Autodesk Inventor part; units mm, degrees
ref_plane "YZ Plane" through (0, 0, 0) normal (1, 0, 0) x (0, 1, 0)
ref_plane "XZ Plane" through (0, 0, 0) normal (0, 1, 0) x (-1, 0, 0)
ref_plane "XY Plane" through (0, 0, 0) normal (0, 0, 1) x (1, 0, 0)
sketch "Sketch1" plane through (0, 0, 0) normal (0, 1, 0) x (-1, 0, 0)
  point P0 (0, 0)
sketch "Sketch2" plane through (0, 0, 0) normal (0, 1, 0) x (-1, 0, 0)
  line L0 (70, -12) -> (70, -66)
  line L1 (70, -66) -> (2, -66)
  line L2 (70, -12) -> (2, -12)
  line L3 (2, -66) -> (2, -12)
  point P0 (0, 0)
  point P1 (2, 0)
  dimension "d151" = 68
  dimension "d152" = 54
extrude "Extrusion1" add sketch "Sketch2" along normal blind 14
sketch "Sketch3" plane through (0, 14, 0) normal (0, 1, 0) x (1, 0, 0)
  point P0 (0, 0)
sketch "Sketch4" plane through (0, 14, 0) normal (0, 1, 0) x (1, 0, 0)
  line L0 (-2, 66) -> (-70, 66)
  line L1 (-30.4814, 66) -> (-28.4814, 66)
  line L2 (-28.4814, 66) -> (-28.4814, 64)
  line L3 (-70, 66) -> (-70, 12)
  line L4 (-70, 37.8423) -> (-70, 39.8423)
  line L5 (-70, 39.8423) -> (-68, 39.8423)
  line L6 (-68, 64) -> (-68, 14)
  line L7 (-68, 64) -> (-4, 64)
  line L8 (-68, 14) -> (-4, 14)
  line L9 (-4, 14) -> (-4, 64)
  line L10 (-70, 12) -> (-2, 12)
  line L11 (-2, 12) -> (-2, 66)
  point P0 (-2, 64)
  point P1 (-68, 12)
  dimension "d6" = 2
  dimension "d8" = 2
  dimension "d102" = 2
  dimension "d104" = 2
  dimension "d153" = 2
  dimension "d154" = 2
extrude "Extrusion2" cut sketch "Sketch4" against normal blind 12 contours L7 L9 L8 L6
sketch "Sketch10" plane through (0, 2, 0) normal (0, 1, 0) x (1, 0, 0)
  line L0 (-48, 14) -> (-48, 17)
  line L1 (-48, 14) -> (-63, 14)
  line L2 (-63, 14) -> (-63, 17)
  line L3 (-63, 17) -> (-48, 17)
  line L4 (-48, 17) -> (-48, 14)
  line L5 (-22, 64) -> (-7, 64)
  line L6 (-7, 64) -> (-7, 61)
  line L7 (-7, 61) -> (-22, 61)
  line L8 (-22, 61) -> (-22, 64)
  line L9 (-68, 64) -> (-4, 64)
  line L10 (-63, 14) -> (-48, 14)
  line L11 (-4, 14) -> (-68, 14)
  point P0 (-68, 2)
  point P1 (-2, 64)
  dimension "d55" = 3
  dimension "d56" = 15
  dimension "d60" = 15
  dimension "d108" = 3
  dimension "d155" = 0
extrude "Extrusion5" add sketch "Sketch10" along normal blind 6
sketch "Sketch12" plane through (0, 0, 0) normal (0, -1, 0) x (1, 0, 0)
  line L0 (0, 0) -> (0, -66)
  arc A0 (-34, -55.9641) -> (-34, -49.0359) centre (-36, -52.5) ccw
  arc A1 (-38, -58.6498) -> (-34, -58.6498) centre (-36, -58.6498) ccw
  line L1 (-34, -58.6498) -> (-34, -55.9641)
  line L2 (-38, -58.6498) -> (-38, -55.9641)
  arc A2 (-34, -49.0359) -> (-38, -55.9641) centre (-36, -52.5) ccw
  line L3 (-2, -12) -> (-2, -66)
  line L4 (-2, -66) -> (-70, -66)
  line L5 (-2, -66) -> (-70, -66)
  line L6 (-36, -66) -> (-36, -12)
  line L7 (-70, -66) -> (-70, -12)
  line L8 (-70, -66) -> (-70, -12)
  line L9 (-70, -39) -> (-2, -39)
  line L10 (-36, -39) -> (-36, -66)
  line L11 (-36, -52.5) -> (-2, -52.5)
  arc A3 (-39, -58.6498) -> (-33, -58.6498) centre (-36, -58.6498) ccw
  line L12 (-39, -58.6498) -> (-39, -56.5)
  arc A4 (-33.5, -48.1699) -> (-39, -56.5) centre (-36, -52.5) ccw
  arc A5 (-33, -56.5) -> (-33.5, -48.1699) centre (-36, -52.5) ccw
  line L13 (-33, -56.5) -> (-33, -58.6498)
  dimension "d156" = 34
  dimension "d157" = 1
extrude "Extrusion7" cut sketch "Sketch12" against normal blind 5 contours L1 A1 L6 L11 A0 | L11 L6 A2 A0 | L6 A1 L2 A2
sketch "Sketch13" plane through (0, 14, 0) normal (0, 1, 0) x (1, 0, 0)
  line L0 (-70, 66) -> (-70, 12)
  line L1 (-69, 65) -> (-69, 13)
  line L2 (-2, 66) -> (-70, 66)
  line L3 (-68, 64) -> (-4, 64)
  line L4 (-2, 64) -> (-2, 12)
  line L5 (-68, 14) -> (-68, 64)
  line L6 (-4, 14) -> (-68, 14)
  line L7 (-68, 14) -> (-4, 14)
  line L8 (-7, 64) -> (-4, 64)
  line L9 (-4, 14) -> (-4, 64)
  line L10 (-70, 12) -> (-2, 12)
  line L11 (-68, 13) -> (-69, 13)
  line L12 (-68, 13) -> (-3, 13)
  line L13 (-2, 12) -> (-2, 66)
  line L14 (-4, 13) -> (-3, 13)
  line L15 (-3, 13) -> (-3, 64)
  line L16 (-3, 64) -> (-3, 65)
  line L17 (-3, 65) -> (-69, 65)
  dimension "d96" = 1
  dimension "d99" = 1
extrude "Extrusion8" cut sketch "Sketch13" against normal blind 2 contours L17 L16 L15 L12 L11 L1 | L3 L9 L6 L5
sketch "Sketch15" plane through (-70, 0, -66) normal (-1, 0, 0) x (0, 0, 1)
  line L0 (62.4242, 8) -> (52.7396, 8)
  line L1 (0, 0) -> (66, 0)
  line L2 (0, 14) -> (54, 14)
  line L3 (0, 0) -> (0, 14)
  line L4 (18.77, 12) -> (27.77, 12)
  line L5 (27.77, 12) -> (27.77, 17)
  line L6 (27.77, 17) -> (18.77, 17)
  line L7 (18.77, 17) -> (18.77, 12)
  point P0 (66, 14)
  dimension "d118" = 8
  dimension "d140" = 27.77
  dimension "d141" = 9
  dimension "d143" = 5
  dimension "d150" = 4
extrude "Extrusion9" cut sketch "Sketch15" against normal blind 10
sketch "Sketch16" plane through (-2, 0, -66) normal (0, 0, -1) x (-1, 0, 0)
  line L0 (39.4, 14) -> (47.9, 14)
  line L1 (47.9, 14) -> (47.9, 9)
  line L2 (47.9, 9) -> (39.4, 9)
  line L3 (39.4, 9) -> (39.4, 14)
  line L4 (54.5, 14) -> (63, 14)
  line L5 (63, 14) -> (63, 9)
  line L6 (63, 9) -> (54.5, 9)
  line L7 (54.5, 9) -> (54.5, 14)
  line L8 (20, 8) -> (5, 8)
  line L9 (68, 0) -> (68, 14)
  point P0 (-2, 0)
  dimension "d127" = 8.5
  dimension "d128" = 8.5
  dimension "d131" = 28.6
  dimension "d132" = 13.5
  dimension "d148" = 5
  dimension "d149" = 6
extrude "Extrusion10" cut sketch "Sketch16" against normal blind 10
fillet "Fillet7" radius 2 1 edges at (-2, 7, -66)
fillet "Fillet8" radius 2 1 edges at (-70, 7, -66)
properties part number "Shell 3 bottom"
Could you check a few things on this model? Use its own coordinates, in mm. A direction names the side the tool comes from. Give positions to 0.01 mm unless a question says otherwise; leave off trailing zeros. Write each loop counter-clockwise with the first axis right and the second up, starting at its lowest first coordinate (ties: lowest second). Pieces come first, ordered by that corner, then holes. Notation, with made-up numbers: (9.5, -20) -> (55.5, -20) arc R17 ccw to (55.5, -15) -> close; hole circle Ø10 at (3.5, 81.25). An arc over 180 degrees is marked (long way). Write each question's results on one line, items separated by ' | '. Start each with the question number.
Q1. I need wall thicknesses on probe 1 along X at (y, z) = (9.5, -52); probe 2 along Z at (x, y) = (-18, 13); probe 3 along Z at (x, y) = (-18, 11). Which ranges of each line are inside material? Lowest first, please.
Q2. Suppose I cut it at C-C, the plane y = 7.25. List the corners of the cut face in (x, z) for me, and give its area (3 significant figures).
Q3. I'm going to push flat-ended pins straight in: pin 1 Ø1 at (x, z) = (-47.5, -64.5) entering from +Y; pin 2 Ø3 at (x, z) = (-39, -50.5) entering from +Y; pin 3 Ø3.5 at (x, z) = (-16, -62) entering from +Y. Where does each tip first touch, or does it pass through?
Q4. Suppose I cut it at D-D, the plane x = -58. List the corners of the cut face in (y, z) for me.
Q5. Suppose I cut it at A-A, the plane z = -52.5. List the corners of the cut face in (x, y) for me, and give its area (3 significant figures).
Q6. Which directions (+Z, -Z, +X, -X, +Y, -Y) give clear straight access to the entire face, cutting with the end or side of a thin tool? Please do faces 3 (the face through (-41.4, 11, -65)), 4 (the face through (-38, 1, -57)), 5 (the face through (-4, 7, -39)).
Q7. We'd pull the mould along X, two halves only. Please class faces 1 (the face through (-36, 7, -66)), 2 (the face through (-36, 2, -39)): +X half, -X half, draft (parallel to the pull), parting line (faces both ways), or undercut.
Q8. Suppose I cut it at B-B, the plane x = -36. List the corners of the cut face in (y, z) for me.
Outcome:
1) probe 1: -70 to -68, -4 to -2 | probe 2: -66 to -65, -13 to -12 | probe 3: -66 to -64, -14 to -12
2) outline: (-70, -64) arc R2 ccw to (-68, -66) -> (-4, -66) arc R2 ccw to (-2, -64) -> (-2, -12) -> (-70, -12) -> close; hole (-68, -64) -> (-22, -64) -> (-22, -61) -> (-7, -61) -> (-7, -64) -> (-4, -64) -> (-4, -14) -> (-48, -14) -> (-48, -17) -> (-63, -17) -> (-63, -14) -> (-68, -14) -> close | area: 560 mm2
3) pin 1: y = 9 | pin 2: y = 2 | pin 3: y = 8
4) outline: (0, -66) -> (9, -66) -> (9, -64) -> (2, -64) -> (2, -17) -> (8, -17) -> (8, -14) -> (12, -14) -> (12, -13) -> (14, -13) -> (14, -12) -> (0, -12) -> close
5) outline: (-70, 0) -> (-40, 0) -> (-40, 2) -> (-68, 2) -> (-68, 12) -> (-69, 12) -> (-69, 14) -> (-70, 14) -> close; (-32, 0) -> (-2, 0) -> (-2, 14) -> (-3, 14) -> (-3, 12) -> (-4, 12) -> (-4, 2) -> (-32, 2) -> close | area: 164 mm2
6) face 3: -Z, +Y | face 4: +Y, -Y | face 5: +Y
7) face 1: draft | face 2: undercut
8) outline: (0, -66) -> (14, -66) -> (14, -65) -> (12, -65) -> (12, -64) -> (2, -64) -> (2, -60.65) -> (0, -60.65) -> close; (0, -48.5) -> (2, -48.5) -> (2, -14) -> (12, -14) -> (12, -13) -> (14, -13) -> (14, -12) -> (0, -12) -> close
